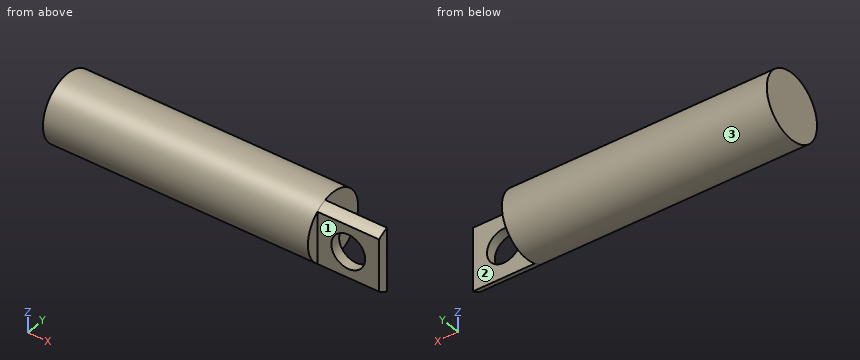
Autodesk Inventor part; units mm, degrees
ref_plane "YZ Plane" through (0, 0, 0) normal (1, 0, 0) x (0, 1, 0)
ref_plane "XZ Plane" through (0, 0, 0) normal (0, 1, 0) x (-1, 0, 0)
ref_plane "XY Plane" through (0, 0, 0) normal (0, 0, 1) x (1, 0, 0)
sketch "Sketch1" plane through (0, 0, 0) normal (1, 0, 0) x (0, 1, 0)
  circle A0 centre (0, 0) radius 8.001
  dimension "d0" = 16.002
extrude "Extrusion1" add sketch "Sketch1" along normal blind 64.3128
sketch "Sketch2" plane through (64.3128, 0, 0) normal (1, 0, 0) x (0, 0, -1)
  line L0 (-6.2432, -5.0038) -> (6.2432, -5.0038)
  line L1 (-7.5991, -2.5038) -> (7.5991, -2.5038)
  arc A0 (6.2432, -5.0038) -> (7.5991, -2.5038) centre (0, 0) ccw
  arc A1 (-7.5991, -2.5038) -> (-6.2432, -5.0038) centre (0, 0) ccw
  circle A2 centre (0, 0) radius 8.001
  point P0 (7.0332, -3.8145)
  point P1 (-7.0332, -3.8145)
  dimension "d3" = 5.0038
  dimension "d4" = 2.5
extrude "Extrusion2" add sketch "Sketch2" along normal blind 15.0114 contours A1 L1 A0 L0
sketch "Sketch3" plane through (64.3128, -2.5038, 7.5991) normal (0, 1, 0) x (1, 0, 0)
  circle A0 centre (7.5057, 7.5991) radius 4.1021
  line L0 (0, 15.1983) -> (15.0114, 15.1983)
  line L1 (0, 0) -> (15.0114, 0)
  point P0 (-64.3128, 7.5991)
  point P1 (7.5057, 15.1983)
  dimension "d8" = 8.2042
  dimension "d9" = 7.5991
  dimension "d10" = 15.1983
extrude "Extrusion3" cut sketch "Sketch3" against normal blind 15.0114
equation "\"d9\" = 0.5 * d10"
properties part number "Ring Connector model 2"
Could you check a few things on this model? Use its own coordinates, in mm. Face numbers are marked on the shaded views. A direction names the side the tool comes from. Coordinates: 2 decimals unless noted, no trailing zeros. Order: outer loops, then holes, each group sorted by start corner. A loop starts at its lowest first (then second) coordinate and runs counter-clockwise, first axis right, second up. Notation, with made-up numbers: (8, 54.5) - (21, 54.5) arc R18 cw to (21, 75.5) - close; hole circle Ø8 at (-31.5, 21.25). An arc over 180 degrees is marked (long way). Answer in a Markdown table with one row per item. Add a question column.
(1) On a 3-axis mill with a long thin cutter (end or side, diameter ignored), from which of +Z, -Z, +X, -X, +Y, -Y can I reach the whole of each face in a straight line? I mean the marked faces 1, 2 and 3. Say none if no direction works.
(2) If we section it at A-A, the plane z = 0: Please give me the cut outline in (x, y), then the cut area to 3 significant figures.
(3) If we section it at C-C, the plane y = 0: Please give me the cut outline in (x, z), then the cut area to 3 significant figures.
(4) I need wall thicknesses on L1, parallel to X at y = -3.9, z = 0; L2, parallel to Y at x = 37, z = 2.5; L3, parallel to Y at x = 71, z = 5.75. Which ranges of each line are inside material? Lowest first, please.
(5) Will these pins go through, and if not, where does the flat tip stop? pin 1 (3 mm diameter, centred on x = 42, y = -5.5, fed in from -Z); pin 2 (0.9 mm diameter, centred on y = -6.5, z = 1, fed in from +X); pin 3 (7.5 mm diameter, centred on x = 69, z = 2.5, fed in from +Y); pin 4 (7.5 mm diameter, centred on x = 71.82, z = 0, fed in from +Y).
(6) If we section it at B-B, the plane x = 6: Please give me the cut outline in (y, z).
(7) If we section it at D-D, the plane z = 3: Please give me the cut outline in (x, y), then the cut area to 3 significant figures.
Results are:
| question | item | result |
|---|---|---|
| 1 | face 1 | +Z, -Z, +X, -Y |
| 1 | face 2 | +Z, -Z, +X, +Y |
| 1 | face 3 | +X, -X |
| 2 | outline | (0, -8) - (64.31, -8) - (64.31, -5) - (67.72, -5) - (67.72, -2.5) - (64.31, -2.5) - (64.31, 8) - (0, 8) - close; (75.92, -5) - (79.32, -5) - (79.32, -2.5) - (75.92, -2.5) - close |
| 2 | area | 1,050 mm2 |
| 3 | outline | (0, -8) - (64.31, -8) - (64.31, 8) - (0, 8) - close |
| 3 | area | 1,030 mm2 |
| 4 | L1 | x = 0 to 67.72, 75.92 to 79.32 |
| 4 | L2 | y = -7.6 to 7.6 |
| 4 | L3 | y = -5 to -2.5 |
| 5 | pin 1 | stops at z = -6.93 |
| 5 | pin 2 | stops at x = 64.31 |
| 5 | pin 3 | stops at y = -2.5 |
| 5 | pin 4 | passes through |
| 6 | outline | circle Ø16 at (0, 0) |
| 7 | outline | (0, -7.42) - (64.31, -7.42) - (64.31, -5) - (69.02, -5) - (69.02, -2.5) - (64.31, -2.5) - (64.31, 7.42) - (0, 7.42) - close; (74.62, -5) - (79.32, -5) - (79.32, -2.5) - (74.62, -2.5) - close |
| 7 | area | 978 mm2 |
